Read the model definition and answer for the solid it produces. Units are mm, in the model's axes. Face numbers are marked on the shaded views. A direction names the side the tool comes from. Coordinates: 2 decimals unless noted, no trailing zeros. Loops run counter-clockwise (first coordinate to the right, second up) from the corner with the lowest first, then second, coordinate; pieces in that order, holes last.
Q1. Section A-A (z = 10.75) is taken. Give the vertices of the cut face in (x, y).
Q2. Which of the six approach directions +Z, -Z, +X, -X, +Y, -Y give full straight-line access (tool end or side, diameter ignored) to the marked faces 1 and 2?
Q3. Section B-B (y = 6.25) is taken. Give the vertices of the cut face in (x, z).
Q4. The mould has two halves that part along X. Classify the marked faces 3, 4, 5 and 6: pulls with the +X half, pulls with the -X half, needs draft (parallel to the pull), parting line crosses it, or undercut.
Q5. Flat-ended cylindrical pins translate along their axes: P1, Ø2.5, axis at x = -21.5, y = 9.5, coming from the +Z side; P2, Ø12.5, axis at x = 17, y = 2.5, coming from the +Z side; P3, Ø3, axis at x = 25, y = -9.5, coming from the +Z side. Find the tip coordinate at first contact, or state that the pin passes through.
Q6. Section D-D (y = 0) is taken. Give the vertices of the cut face in (x, z), then the cut area to 3 significant figures.
Q7. Straight lines are drawn through the part: line 1 (Y direction, x = -11, z = 11.5); line 2 (X direction, y = -2.75, z = 6.25); line 3 (Y direction, x = 24, z = 5.75). For each, find the intervals that lie inside material, in ascending order.
Q8. Section C-C (x = 3.5) is taken. Give the vertices of the cut face in (y, z).
from build123d import *

# Parameters (mm, degrees)
F1_DEPTH  = 13.97
F2_T      = -1.27
F3_R      = 2.032
F3_R_2    = 0.8255
F4_DEPTH  = 3.81
F5_DEPTH  = 5.461
F6_DEPTH  = 2.54
F7_W      = 8.89
F7_H      = 3.1753103511
F7_W_2    = 5.08
F7_H_2    = 2.7178
F8_DEPTH  = 1.905
F9_R      = 0.9525
F10_DEPTH = 1.905
F11_R     = 2.032
F11_R_2   = 0.8255
F12_DEPTH = 3.81
F14_DEPTH = 2.032
F15_W     = 3.3083129674
F15_H     = 4.001185298
F15_W_2   = 4.9948431551
F15_H_2   = 3.4223934636
F15_W_3   = 4.9023460597
F15_H_3   = 4.0236227214
F16_DEPTH = 1.27


with BuildPart() as f1:
    # F0 (on Top) → F1 (new body)
    with BuildSketch(Plane.XY):
        with BuildLine():
            Line((-21.5788040441, -13.9683183577), (29.7179990722, -13.9683183577))
            ThreePointArc((29.7179990722, -13.9683183577), (32.4120759085, -12.852395194), (33.5279990722, -10.1583183577))
            Line((33.5279990722, -10.1583183577), (33.5279990722, 9.5266816423))
            ThreePointArc((33.5279990722, 9.5266816423), (32.4120759085, 12.2207584786), (29.7179990722, 13.3366816423))
            Line((29.7179990722, 13.3366816423), (-21.60052527, 13.3366816423))
            ThreePointArc((-21.60052527, 13.3366816423), (-24.2960880723, 12.2192716925), (-25.4105229505, 9.5224775366))
            Line((-25.4105229505, 9.5224775366), (-25.3888017246, -10.1625224634))
            ThreePointArc((-25.3888017246, -10.1625224634), (-24.2713940943, -12.8538811601), (-21.5788040441, -13.9683183577))
        make_face()
    extrude(amount=F1_DEPTH)

    # F2
    f2_openings = [f1.faces().sort_by_distance(p)[0] for p in [
        (4.064166, -0.31477, 13.97),
    ]]
    offset(amount=F2_T, openings=f2_openings)

    # F3 (on face) → F4 (join)
    with BuildSketch(Plane.XY.offset(1.27)):
        with Locations((-21.3360009278, 8.8916816423)):
            Circle(F3_R)
        with Locations((-21.3360009278, 8.8916816423)):
            Circle(F3_R_2, mode=Mode.SUBTRACT)
        with Locations((-21.3360009278, -8.8883183577)):
            Circle(F3_R)
        with Locations((-21.3360009278, -8.8883183577)):
            Circle(F3_R_2, mode=Mode.SUBTRACT)
        with BuildLine():
            Line((26.9239990722, -8.8883183577), (25.5269990722, -8.8883183577))
            ThreePointArc((25.5269990722, -8.8883183577), (24.3839990722, -10.0313183577), (23.2409990722, -8.8883183577))
            Line((23.2409990722, -8.8883183577), (21.8439990722, -8.8883183577))
            ThreePointArc((21.8439990722, -8.8883183577), (24.3839990722, -11.4283183577), (26.9239990722, -8.8883183577))
        make_face()
        with BuildLine():
            ThreePointArc((23.2409990722, 8.8916816423), (24.3839990722, 10.0346816423), (25.5269990722, 8.8916816423))
            Line((25.5269990722, 8.8916816423), (26.9239990722, 8.8916816423))
            ThreePointArc((26.9239990722, 8.8916816423), (24.3839990722, 11.4316816423), (21.8439990722, 8.8916816423))
            Line((21.8439990722, 8.8916816423), (23.2409990722, 8.8916816423))
        make_face()
    extrude(amount=F4_DEPTH)

    # F3 (on face) → F5 (join)
    with BuildSketch(Plane.XY.offset(1.27)):
        with BuildLine():
            Line((24.3839990722, 8.8916816423), (25.5269990722, 8.8916816423))
            ThreePointArc((25.5269990722, 8.8916816423), (24.3839990722, 10.0346816423), (23.2409990722, 8.8916816423))
            Line((23.2409990722, 8.8916816423), (24.3839990722, 8.8916816423))
        make_face()
        with BuildLine():
            ThreePointArc((23.2409990722, 8.8916816423), (24.3839990722, 7.7486816423), (25.5269990722, 8.8916816423))
            Line((25.5269990722, 8.8916816423), (24.3839990722, 8.8916816423))
            Line((24.3839990722, 8.8916816423), (23.2409990722, 8.8916816423))
        make_face()
        with BuildLine():
            Line((24.3839990722, -8.8883183577), (25.5269990722, -8.8883183577))
            ThreePointArc((25.5269990722, -8.8883183577), (24.3839990722, -7.7453183577), (23.2409990722, -8.8883183577))
            Line((23.2409990722, -8.8883183577), (24.3839990722, -8.8883183577))
        make_face()
        with BuildLine():
            ThreePointArc((23.2409990722, -8.8883183577), (24.3839990722, -10.0313183577), (25.5269990722, -8.8883183577))
            Line((25.5269990722, -8.8883183577), (24.3839990722, -8.8883183577))
            Line((24.3839990722, -8.8883183577), (23.2409990722, -8.8883183577))
        make_face()
    extrude(amount=F5_DEPTH)

    # F3 (on face) → F6 (cut)
    with BuildSketch(Plane.XY.offset(1.27)):
        with Locations((-21.3360009278, 8.8916816423)):
            Circle(F3_R_2)
        with Locations((-21.3360009278, -8.8883183577)):
            Circle(F3_R_2)
    extrude(amount=F6_DEPTH, mode=Mode.SUBTRACT)

    # F7 (on face) → F8 (cut)
    with BuildSketch(Plane(origin=(-25.3999845367, -0.0280273712, 0), x_dir=(0.0011034398, -0.9999993912, 0), z_dir=(-0.9999993912, -0.0011034398, 0))):
        with Locations((0, 3.81)):
            Rectangle(F7_W, F7_H)
        with Locations((0, 8.0265551756)):
            Rectangle(F7_W_2, F7_H_2)
    extrude(amount=-F8_DEPTH, mode=Mode.SUBTRACT)

    # F9 (on face) → F10 (cut)
    with BuildSketch(Plane.YZ.offset(33.5279990722)):
        with Locations((5.9706816423, 2.794)):
            Circle(F9_R)
    extrude(amount=-F10_DEPTH, mode=Mode.SUBTRACT)

    # F11 (on face) → F12 (join)
    with BuildSketch(Plane.XY.offset(1.27)):
        with Locations((29.4639990722, 0)):
            Circle(F11_R)
        with Locations((29.4639990722, 0)):
            Circle(F11_R_2, mode=Mode.SUBTRACT)
    extrude(amount=F12_DEPTH)

    # F13 (on face) → F14 (join)
    with BuildSketch(Plane.XY.offset(1.27)):
        with BuildLine():
            ThreePointArc((-14.0236731965, -12.6983183577), (-16.3756129487, -11.7037291087), (-17.9839668508, -9.7202911598))
            Line((-17.9839668508, -9.7202911598), (-18.9684356708, -10.3109590834))
            ThreePointArc((-18.9684356708, -10.3109590834), (-18.1080100407, -11.6293001054), (-16.9523477667, -12.6983183577))
            Line((-16.9523477667, -12.6983183577), (-14.0236731965, -12.6983183577))
        make_face()
        with BuildLine():
            ThreePointArc((-12.3923286591, -12.6983183577), (-13.2080009278, -12.7618183577), (-14.0236731965, -12.6983183577))
            Line((-14.0236731965, -12.6983183577), (-16.9523477667, -12.6983183577))
            ThreePointArc((-16.9523477667, -12.6983183577), (-13.2080009278, -13.9048183577), (-9.4636540889, -12.6983183577))
            Line((-9.4636540889, -12.6983183577), (-12.3923286591, -12.6983183577))
        make_face()
        with BuildLine():
            ThreePointArc((-16.6064980594, -3.4628710766), (-8.4130955389, -5.303384958), (-12.3923286591, -12.6983183577))
            Line((-12.3923286591, -12.6983183577), (-9.4636540889, -12.6983183577))
            ThreePointArc((-9.4636540889, -12.6983183577), (-8.145657173, -3.5535959249), (-17.3335159362, -2.5808083877))
            Line((-17.3335159362, -2.5808083877), (-16.6064980594, -3.4628710766))
        make_face()
    extrude(amount=F14_DEPTH)

    # F15 (on face) → F16 (join)
    with BuildSketch(Plane.XY.offset(1.27)):
        with Locations((31.0986405239, -0.0055211131)):
            Rectangle(F15_W, F15_H)
        with Locations((-21.7511262745, 10.4752979241)):
            Rectangle(F15_W_2, F15_H_2)
        with Locations((-21.7973748222, -10.8221620321)):
            Rectangle(F15_W_3, F15_H_3)
    extrude(amount=F16_DEPTH)


solid = f1.part
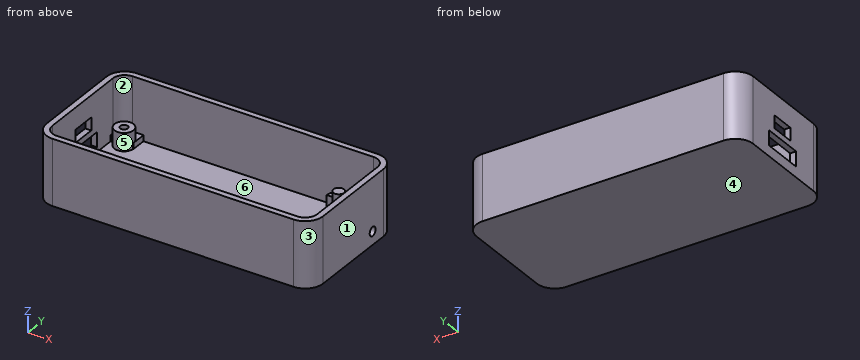
Numbers:
1. outline: (-25.41, 9.52) - (-25.39, -10.16) arc R3.81 ccw to (-21.58, -13.97) - (29.72, -13.97) arc R3.81 ccw to (33.53, -10.16) - (33.53, 9.53) arc R3.81 ccw to (29.72, 13.34) - (-21.6, 13.34) arc R3.81 ccw to start; hole (-24.14, 9.52) - (-24.12, -10.16) arc R2.54 ccw to (-21.58, -12.7) - (29.72, -12.7) arc R2.54 ccw to (32.26, -10.16) - (32.26, 9.53) arc R2.54 ccw to (29.72, 12.07) - (-21.6, 12.07) arc R2.54 ccw to start
2. face 1: +Z, -Z, +X, +Y, -Y
2. face 2: +Z
3. outline: (-25.41, 0) - (33.53, 0) - (33.53, 1.88) - (32.26, 1.88) - (32.26, 1.27) - (-24.14, 1.27) - (-24.14, 13.97) - (-25.41, 13.97) - close; (32.26, 3.7) - (33.53, 3.7) - (33.53, 13.97) - (32.26, 13.97) - close
4. face 3: pulls with the +X half
4. face 4: needs draft
4. face 5: undercut
4. face 6: undercut
5. P1: stops at z = 5.08
5. P2: stops at z = 1.27
5. P3: stops at z = 6.73
6. outline: (-25.4, 0) - (33.53, 0) - (33.53, 13.97) - (32.26, 13.97) - (32.26, 2.54) - (31.5, 2.54) - (31.5, 5.08) - (30.29, 5.08) - (30.29, 2.54) - (29.44, 2.54) - (29.44, 1.27) - (28.64, 1.27) - (28.64, 5.08) - (27.43, 5.08) - (27.43, 1.27) - (-24.13, 1.27) - (-24.13, 2.22) - (-25.4, 2.22) - close; (-25.4, 5.4) - (-24.13, 5.4) - (-24.13, 6.67) - (-25.4, 6.67) - close; (-25.4, 9.39) - (-24.13, 9.39) - (-24.13, 13.97) - (-25.4, 13.97) - close
6. area: 111 mm2
7. line 1: y = -13.97 to -12.7, 12.07 to 13.34
7. line 2: x = -25.4 to -24.13, 32.26 to 33.53
7. line 3: y = -13.97 to -12.7, -9.96 to -7.81, 7.82 to 9.97, 12.07 to 13.34
8. outline: (-13.97, 0) - (13.34, 0) - (13.34, 13.97) - (12.07, 13.97) - (12.07, 1.27) - (-12.7, 1.27) - (-12.7, 13.97) - (-13.97, 13.97) - close
